from build123d import *

# Parameters (mm, degrees)
SKETCH_1_R      = 125
EXTRUDE_1_DEPTH = 15
SKETCH_2_R      = 108.5
EXTRUDE_2_DEPTH = 330
SKETCH_4_W      = 50
SKETCH_4_H      = 70
EXTRUDE_4_DEPTH = 200
SKETCH_6_R      = 100
EXTRUDE_5_DEPTH = 50
SKETCH_7_R      = 100
EXTRUDE_6_DEPTH = 50


with BuildPart() as part:
    # 草图1 → 凸台-拉伸1 (new body)
    with BuildSketch(Plane.XY):
        Circle(SKETCH_1_R)
    extrude(amount=EXTRUDE_1_DEPTH)

    # 草图2 → 凸台-拉伸2 (add)
    with BuildSketch(Plane.XY.offset(15)):
        Circle(SKETCH_2_R)
    extrude(amount=EXTRUDE_2_DEPTH)

    # 草图4 → 旋转1 (revolve)
    with BuildSketch(Plane.XY.offset(220)):
        with Locations((-25, 131.292523074)):
            Rectangle(SKETCH_4_W, SKETCH_4_H)
    revolve(axis=Axis((0, 165.766992941, 220), (0, -1, 0)))

    # 草图5 → 凸台-拉伸4 (add)
    with BuildSketch(Plane(origin=(0, 0, 0), x_dir=(-1, 0, 0), z_dir=(0, 0, -1))):
        with BuildLine():
            Line((-73.496377584, 101.110249144), (73.496377584, 101.110249144))
            ThreePointArc((73.496377584, 101.110249144), (111.382330731, 56.736023838), (125, 0))
            Line((125, 0), (125, -375))
            Line((125, -375), (-125, -375))
            Line((-125, -375), (-125, 0))
            ThreePointArc((-125, 0), (-111.382330731, 56.736023838), (-73.496377584, 101.110249144))
        make_face()
    extrude(amount=EXTRUDE_4_DEPTH)

    # 草图6 → 凸台-拉伸5 (add)
    with BuildSketch(Plane(origin=(0, 0, -200), x_dir=(-1, 0, 0), z_dir=(0, 0, -1))):
        with Locations((0, -250)):
            Circle(SKETCH_6_R)
    extrude(amount=EXTRUDE_5_DEPTH)

    # 草图7 → 凸台-拉伸6 (add)
    with BuildSketch(Plane.XY):
        with Locations((0, -250)):
            Circle(SKETCH_7_R)
    extrude(amount=EXTRUDE_6_DEPTH)


solid = part.part
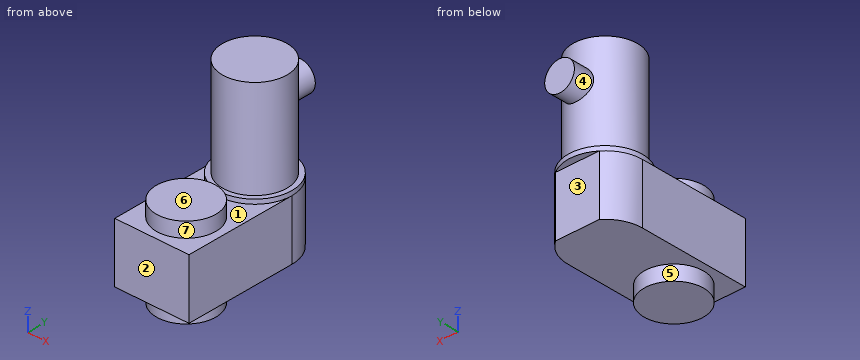
Build history of the part. All positions in model axes, mm. Face numbers are marked on the shaded views. A direction names the side the tool comes from. Round coordinates to 2 decimals unless told otherwise and drop trailing zeros. Write each loop counter-clockwise with the first axis right and the second up, starting at its lowest first coordinate (ties: lowest second). Pieces come first, ordered by that corner, then holes. Notation, with made-up numbers: M -30.5,31 L 22.5,31 A24 ccw 22.5,66 Z; hole C -6,42 d10. An arc over 180 degrees is marked long. Answer in a Markdown table with one row per item.
1. Flat gauge pins, fed straight in: P1, Ø7, axis at x = 23, y = 107, coming from the -Z side; P2, Ø1.5, axis at y = 34.5, z = 49, coming from the -X side; P3, Ø3, axis at x = 53, z = 230, coming from the +Y side. Where does each tip first touch, or does it go through?
Geometry check:
| item | result |
|---|---|
| P1 | z = 0 |
| P2 | x = -103.12 |
| P3 | y = 95.5 |
2. Which spindle directions (+Z, -Z, +X, -X, +Y, -Y) get a long thin tool onto all of the face, cutting with end or side? Do the marked faces 4, 5, 6 and 7. Say none if no direction does.
Geometry check:
| item | result |
|---|---|
| face 4 | +Y |
| face 5 | -Z |
| face 6 | +Z, +X, -X, -Y |
| face 7 | +Z |
3. Mould opens along Y. For the marked faces 1, 2 and 3 say: +Y half, -Y half, draft (parallel to the pull), parting line (faces both ways), or undercut.
Geometry check:
| item | result |
|---|---|
| face 1 | undercut |
| face 2 | -Y half |
| face 3 | +Y half |
4. Saw through at A-A (x = 22.5). List the corners of the cut face in (y, z).
Geometry check:
| item | result |
|---|---|
| outline | M -375,-200 L -347.44,-200 L -347.44,-250 L -152.56,-250 L -152.56,-200 L 101.11,-200 L 101.11,0 L 122.96,0 L 122.96,15 L 106.14,15 L 106.14,175.35 L 166.29,175.35 L 166.29,264.65 L 106.14,264.65 L 106.14,345 L -106.14,345 L -106.14,15 L -122.96,15 L -122.96,0 L -152.56,0 L -152.56,50 L -347.44,50 L -347.44,0 L -375,0 Z |
5. Saw through at D-D (x = -31). List the corners of the cut face in (y, z) (3 decimals), and give its area (3 significant figures).
Geometry check:
| item | result |
|---|---|
| outline | M -375,-200 L -345.074,-200 L -345.074,-250 L -154.926,-250 L -154.926,-200 L 101.11,-200 L 101.11,0 L 121.095,0 L 121.095,15 L 103.977,15 L 103.977,180.77 L 166.293,180.77 L 166.293,259.23 L 103.977,259.23 L 103.977,345 L -103.977,345 L -103.977,15 L -121.095,15 L -121.095,0 L -154.926,0 L -154.926,50 L -345.074,50 L -345.074,0 L -375,0 Z |
| area | 191,000 mm2 |
6. Probe L1, parallel to Z at x = -48, y = -320; L2, parallel to Z at x = 68, y = 24; L3, parallel to X at y = 3.5, z = 157.5. List the from-to ranges inside material, lowest first. Write a range as [from, to].
Geometry check:
| item | result |
|---|---|
| L1 | [-250, 50] |
| L2 | [-200, 345] |
| L3 | [-108.44, 108.44] |
7. Saw through at B-B (y = -250). List the corners of the cut face in (x, z).
Geometry check:
| item | result |
|---|---|
| outline | M -125,-200 L -100,-200 L -100,-250 L 100,-250 L 100,-200 L 125,-200 L 125,0 L 100,0 L 100,50 L -100,50 L -100,0 L -125,0 Z |
8. Saw through at C-C (z = -21.5). List the corners of the cut face in (x, y), and give its area (3 significant figures).
Geometry check:
| item | result |
|---|---|
| outline | M -125,-375 L 125,-375 L 125,0 A125 ccw 73.5,101.11 L -73.5,101.11 A125 ccw -125,0 Z |
| area | 116,000 mm2 |
